Solid Edge part; units mm, degrees
sketch "Sketch1" plane through (0, 0, 0) normal (0, 0, 1) x (1, 0, 0)
  line L0 (30, 75) -> (30, 30)
  line L1 (30, 30) -> (60, 30)
  line L2 (60, 30) -> (60, 75)
  line L3 (60, 75) -> (30, 75)
  line L4 (120, 30) -> (0, 30)
  line L5 (0, 30) -> (0, 0)
  line L6 (0, 0) -> (120, 0)
  line L7 (120, 0) -> (120, 30)
extrude "Protrusion1" add sketch "Sketch1" along normal blind 4
fillet "RoundMain" radius 15 6 edges at (0, 30, 2) (30, 75, 2) (60, 75, 2) (120, 30, 2) (120, 0, 2) (0, 0, 2)
sketch "Sketch2" plane through (60, 37.5, 0) normal (0, 0, -1) x (-1, 0, 0)
  line L0 (0, -7.5) -> (-2, -7.5)
  line L1 (-2, -7.5) -> (-2, -37.5)
  line L2 (-2, -37.5) -> (0, -37.5)
  line L3 (0, -37.5) -> (0, -7.5)
extrude "ExtrudedProtrusion_3" add sketch "Sketch2" along normal blind 1
sketch "Sketch3" plane through (30, 37.5, 0) normal (0, 0, -1) x (-1, 0, 0)
  line L0 (-28.9101, -7.5) -> (-21.9101, -7.5)
  line L1 (-21.9101, -7.5) -> (-21.9101, -5.4965)
  line L2 (-21.9101, -5.4965) -> (-28.9101, -5.4965)
  line L3 (-28.9101, -5.4965) -> (-28.9101, -7.5)
extrude "ExtrudedProtrusion_6" add sketch "Sketch3" along normal blind 1
Read the model definition and answer for the solid it produces. Units are mm, in the model's axes. A direction names the side the tool comes from. Give positions to 0.01 mm unless a question says otherwise; leave off trailing zeros. Loops run counter-clockwise (first coordinate to the right, second up) from the corner with the lowest first, then second, coordinate; pieces in that order, holes last.
Item 1: For faces 1 (the flat face through (30, 45, 2)), 2 (the flat face through (59, 30, 4)), 3 (the flat face through (60, 45, 2)), 4 (the flat face through (91, 15, 0)), determine the directions among +Z, -Z, +X, -X, +Y, -Y from which every point of the face is accessible in a straight line to the end or side of a thin tool.
Item 2: The part is cut by section B-B (y = 10). Write down the section's boundary in (x, z).
Item 3: Each of these flat-tipped pins is pushed along its axis until it touches: pin 1 Ø0.8 at (y, z) = (31.5, -0.5) entering from +X; pin 2 Ø12 at (x, y) = (67.5, 63.5) entering from -Z; pin 3 Ø3 at (y, z) = (38.5, 1.5) entering from +X; pin 4 Ø5 at (x, y) = (39.5, 10) entering from -Z. Where does it stop, or does it pass through?
Item 4: The part is cut by section C-C (x = 94.5). Write down the section's boundary in (y, z), and give its area (3 significant figures).
Item 5: The part is cut by section D-D (y = 38.5). Write down the section's boundary in (x, z).
Item 6: Find the intervals of material crossed by line 1 along X through (y, z) = (44, 0.85); line 2 along Z through (x, y) = (7, 3); line 3 along X through (y, z) = (26, -0.2), in increasing order.
Taken from the geometry:
1. face 1: +Z, -Z, -X, +Y
1. face 2: +Z, +X, -X, +Y, -Y
1. face 3: +Z, -Z, +X, +Y
1. face 4: -Z, +X, +Y, -Y
2. outline: (0.86, 0) - (60, 0) - (60, -1) - (62, -1) - (62, 0) - (119.14, 0) - (119.14, 4) - (0.86, 4) - close
3. pin 1: stops at x = 58.91
3. pin 2: passes through
3. pin 3: stops at x = 60
3. pin 4: stops at z = 0
4. outline: (0, 0) - (30, 0) - (30, 4) - (0, 4) - close
4. area: 120 mm2
5. outline: (30, 0) - (60, 0) - (60, 4) - (30, 4) - close
6. line 1: x = 30 to 60
6. line 2: z = 0 to 4
6. line 3: x = 60 to 62
